Check sheet for the modelled part. Datum: model origin and axes. Units: mm. Face numbers are marked on the shaded views. Round coordinates to 2 decimals unless told otherwise and drop trailing zeros. Write each loop counter-clockwise with the first axis right and the second up, starting at its lowest first coordinate (ties: lowest second). Pieces come first, ordered by that corner, then holes. Notation, with made-up numbers: (30, -28) -> (61, -28) arc R12 ccw to (61, -11) -> close; hole circle Ø7 at (46, 89.5). An arc over 180 degrees is marked (long way). Write item = value, one per line.
from build123d import *

# Parameters (mm, degrees)
ESQUISSE1_W        = 55
ESQUISSE1_H        = 60
ESQUISSE1_R        = 17
ESQUISSE1_W_2      = 5
ESQUISSE1_H_2      = 5
ESQUISSE1_H_3      = 10
BOSS_EXTRU_1_DEPTH = 5


with BuildPart() as part:
    # Esquisse1 → Boss.-Extru.1 (new body)
    with BuildSketch(Plane.XY):
        with Locations((27.5, 30)):
            Rectangle(ESQUISSE1_W, ESQUISSE1_H)
        with Locations((27.5, 30)):
            Circle(ESQUISSE1_R, mode=Mode.SUBTRACT)
        with Locations((12.5, 62.5)):
            Rectangle(ESQUISSE1_W_2, ESQUISSE1_H_2)
        with Locations((2.5, 62.5)):
            Rectangle(ESQUISSE1_W_2, ESQUISSE1_H_2)
        with Locations((22.5, 62.5)):
            Rectangle(ESQUISSE1_W_2, ESQUISSE1_H_2)
        with Locations((32.5, 62.5)):
            Rectangle(ESQUISSE1_W_2, ESQUISSE1_H_2)
        with Locations((52.5, 62.5)):
            Rectangle(ESQUISSE1_W_2, ESQUISSE1_H_2)
        with Locations((42.5, 62.5)):
            Rectangle(ESQUISSE1_W_2, ESQUISSE1_H_2)
        with Locations((2.5, -5)):
            Rectangle(ESQUISSE1_W_2, ESQUISSE1_H_3)
        with Locations((12.5, -5)):
            Rectangle(ESQUISSE1_W_2, ESQUISSE1_H_3)
        with Locations((22.5, -5)):
            Rectangle(ESQUISSE1_W_2, ESQUISSE1_H_3)
        with Locations((32.5, -5)):
            Rectangle(ESQUISSE1_W_2, ESQUISSE1_H_3)
        with Locations((42.5, -5)):
            Rectangle(ESQUISSE1_W_2, ESQUISSE1_H_3)
        with Locations((52.5, -5)):
            Rectangle(ESQUISSE1_W_2, ESQUISSE1_H_3)
    extrude(amount=BOSS_EXTRU_1_DEPTH)


solid = part.part
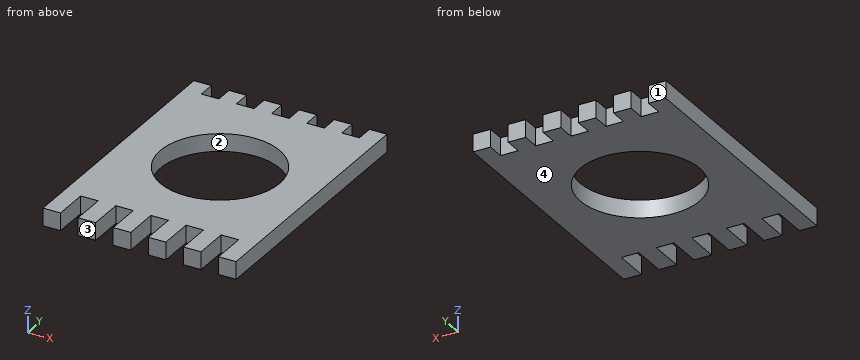
(1) Sectioned sample at B-B on y = 30. Enter the section's corners in (x, z).
Worked answers:
outline = (0, 0) -> (10.5, 0) -> (10.5, 5) -> (0, 5) -> close; (44.5, 0) -> (55, 0) -> (55, 5) -> (44.5, 5) -> close
(2) Material ranges on L1, parallel to Y at x = 27.5, z = 3.85; L2, parallel to X at y = 62.5, z = 3.4; L3, parallel to Y at x = 21.5, z = 4.15, recorded low to high. Write a range as [from, to].
Worked answers:
L1 = [0, 13], [47, 60]
L2 = [0, 5], [10, 15], [20, 25], [30, 35], [40, 45], [50, 55]
L3 = [-10, 14.09], [45.91, 65]
(3) Go/stop test with flat-tipped pins: P1, Ø1.5, axis at x = 46, z = 1, coming from the -Y side; P2, Ø1.5, axis at x = 18, z = 3.5, coming from the +Y side. Record where each tip stops, or that it passes through.
Worked answers:
P1 = 0
P2 = 60
(4) Sectioned sample at A-A on x = 27.5. Enter the section's corners in (y, z).
Worked answers:
outline = (0, 0) -> (13, 0) -> (13, 5) -> (0, 5) -> close; (47, 0) -> (60, 0) -> (60, 5) -> (47, 5) -> close
(5) Sectioned sample at C-C on x = 48. Enter the section's corners in (y, z), then the cut area to 3 significant figures.
Worked answers:
outline = (0, 0) -> (60, 0) -> (60, 5) -> (0, 5) -> close
area = 300 mm²
(6) Release check for a two-part mould opening along Y. For the marked faces 1, 2, 3 and 4 record: pulls with the +Y half, pulls with the -Y half, needs draft (parallel to the pull), parting line crosses it, or undercut.
Worked answers:
face_1 = pulls with the +Y half
face_2 = undercut
face_3 = pulls with the -Y half
face_4 = needs draft
